```python
from build123d import *

# Parameters (mm, degrees)
BOSS_EXTRUDE1_DEPTH = 5
BOSS_EXTRUDE2_DEPTH = 5
BOSS_EXTRUDE3_DEPTH = 5
CIRPATTERN1_COUNT   = 12
CIRPATTERN2_COUNT   = 27


with BuildPart() as part:
    # Sketch1 → Boss-Extrude1 (new, symmetric)
    # profile 1 of 3: a face of its own
    with BuildSketch(Plane(origin=(0, 0, 0), x_dir=(-1, 0, 0), z_dir=(0, 1, 0))):
        with BuildLine():
            ThreePointArc((15, 0), (14.987975919, 0.600481349), (14.951922953, 1.2))
            ThreePointArc((14.951922953, 1.2), (-15, 0), (14.951922953, -1.2))
            ThreePointArc((14.951922953, -1.2), (14.987975919, -0.600481349), (15, 0))
        make_face()
        with BuildLine():
            Line((-1, 9.949874371), (-1, 10))
            Line((-1, 10), (0, 10))
            Line((0, 10), (1, 10))
            Line((1, 10), (1, 9.949874371))
            ThreePointArc((1, 9.949874371), (7.416198487, 6.708203932), (10, 0))
            ThreePointArc((10, 0), (-6.708203932, -7.416198487), (-1, 9.949874371))
        make_face(mode=Mode.SUBTRACT)
    # profile 2 of 3: a face of its own
    with BuildSketch(Plane(origin=(0, 0, 0), x_dir=(-1, 0, 0), z_dir=(0, 1, 0))):
        with BuildLine():
            Line((1, 10), (0, 10))
            ThreePointArc((0, 10), (0.500627751, 9.987460731), (1, 9.949874371))
            Line((1, 9.949874371), (1, 10))
        make_face()
    # profile 3 of 3: a face of its own
    with BuildSketch(Plane(origin=(0, 0, 0), x_dir=(-1, 0, 0), z_dir=(0, 1, 0))):
        with BuildLine():
            Line((0, 10), (-1, 10))
            Line((-1, 10), (-1, 9.949874371))
            ThreePointArc((-1, 9.949874371), (-0.500627751, 9.987460731), (0, 10))
        make_face()
    extrude(amount=BOSS_EXTRUDE1_DEPTH, both=True)

    # Sketch1_3 → Boss-Extrude2 (add, symmetric)
    with BuildSketch(Plane(origin=(0, 0, 0), x_dir=(-1, 0, 0), z_dir=(0, 1, 0))):
        with BuildLine():
            ThreePointArc((17.989997221, -0.6), (18, 0), (17.989997221, 0.6))
            Line((17.989997221, 0.6), (14.951922953, 1.2))
            ThreePointArc((14.951922953, 1.2), (14.987975919, 0.600481349), (15, 0))
            ThreePointArc((15, 0), (14.987975919, -0.600481349), (14.951922953, -1.2))
            Line((14.951922953, -1.2), (17.989997221, -0.6))
        make_face()
    boss_extrude2 = extrude(amount=BOSS_EXTRUDE2_DEPTH, both=True)

    # Sketch1_4 → Boss-Extrude3 (add, symmetric)
    with BuildSketch(Plane(origin=(0, 0, 0), x_dir=(-1, 0, 0), z_dir=(0, 1, 0))):
        with BuildLine():
            ThreePointArc((1, 9.949874371), (0.500627751, 9.987460731), (0, 10))
            ThreePointArc((0, 10), (-0.500627751, 9.987460731), (-1, 9.949874371))
            Line((-1, 9.949874371), (-1, 9))
            Line((-1, 9), (1, 9))
            Line((1, 9), (1, 9.949874371))
        make_face()
    boss_extrude3 = extrude(amount=BOSS_EXTRUDE3_DEPTH, both=True)

    # CirPattern1: Boss-Extrude3 ×12 about axis
    cirpattern1_axis = Axis((0, 0, 0), (0, 1, 0))
    for i in range(1, CIRPATTERN1_COUNT):
        add(boss_extrude3.rotate(cirpattern1_axis, i * 360 / CIRPATTERN1_COUNT))

    # CirPattern2: Boss-Extrude2 ×27 about axis
    cirpattern2_axis = Axis((0, 0, 0), (0, 1, 0))
    for i in range(1, CIRPATTERN2_COUNT):
        add(boss_extrude2.rotate(cirpattern2_axis, i * 360 / CIRPATTERN2_COUNT))


solid = part.part
```
Geometry: final body of the model. Coordinates: model frame, mm. A direction names the side the tool comes from. Round coordinates to 2 decimals unless told otherwise and drop trailing zeros. Use one line per item in the form item = value. Start each with the question number.
1) Access query for faces 4 (the flat face through (-1.966, 0.07, -16.357)), 5 (the flat face through (-13.2, 0.1, -9.9)), 6 (the flat face through (14.271, 0.07, 8.314)), 7 (the flat face through (-12.02, 0.07, -11.266)). Directions: +Z, -Z, +X, -X, +Y, -Y. A direction counts if a zero-diameter tool reaches every point of the face in a straight line with its end or side. Return the directions, or none.
2) First-contact query: P1, Ø0.8, axis at y = -2.5, z = -9.5, coming from the -X side; P2, Ø0.5, axis at x = 9.5, y = 2, coming from the -Z side; P3, Ø1.6, axis at x = 0, y = -1, coming from the +Z side; P4, Ø4, axis at y = -3, z = -5.5, coming from the +X side. Flat tips, straight axial feed; report the tip coordinate or a pass-through.
3) Line query: L1, parallel to X at y = 0.75, z = 16; L2, parallel to X at y = -2.75, z = -13; L3, parallel to Z at x = 14, y = -4.25. Output: solid intervals per line, ascending.
4) Draft query along X for faces 1 (the cylindrical face through (5.154, 0.07, 17.246)), 2 (the flat face through (7.79, 0.07, -4.51)), 3 (the flat face through (-8.3, 5, 4.3)). Return one class per face: released by +X, released by -X, zero draft, split by the parting line, or undercut.
Response:
q1.face_4 = -Z, +Y, -Y
q1.face_5 = -X, +Y, -Y
q1.face_6 = +X, +Y, -Y
q1.face_7 = +Y, -Y
q2.P1 = -13.2
q2.P2 = -15.44
q2.P3 = 17.99
q2.P4 = 17.11
q3.L1 = -7.62 to -6.05, -3.75 to -1.83, -0.07 to 1.91, 3.84 to 5.63
q3.L2 = -10.71 to -8.29, -7.48 to 8.74, 11.21 to 12.45
q3.L3 = -10.1 to -8.05, -6.3 to 6.3, 8.05 to 10.1
q4.face_1 = released by +X
q4.face_2 = undercut
q4.face_3 = zero draft
